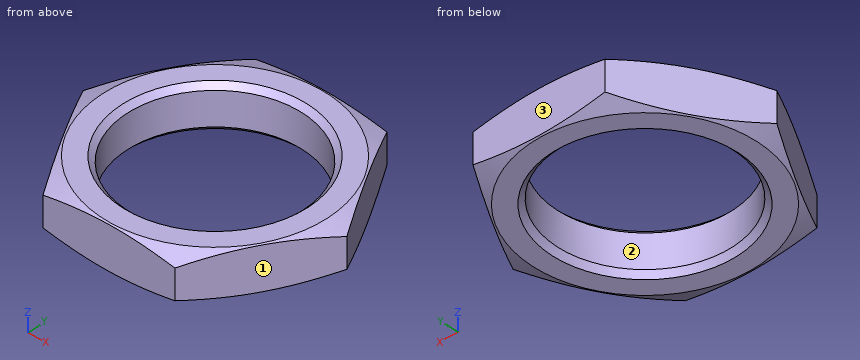
from build123d import *

# Parameters (mm, degrees)
ESQUISSE1_R        = 5
BOSS_EXTRU_1_DEPTH = 2.5
CHANFREIN1_SIZE    = 0.3


with BuildPart() as part:
    # Esquisse1 → Boss.-Extru.1 (new body)
    with BuildSketch(Plane.XY):
        Polygon((7.505553499, 0), (3.75277675, 6.5), (-3.75277675, 6.5), (-7.505553499, 0), (-3.75277675, -6.5), (3.75277675, -6.5), align=None)
        Circle(ESQUISSE1_R, mode=Mode.SUBTRACT)
    extrude(amount=BOSS_EXTRU_1_DEPTH)

    # Esquisse2 → Enlèvement de matière-Révolution1 (revolve, cut)
    with BuildSketch(Plane(origin=(0, 0, 0), x_dir=(1, 0, 0), z_dir=(0, 1, 0))):
        Polygon((-6.405553499, 0), (-7.505553499, -0.400367258), (-7.505553499, -2.099632742), (-6.405553499, -2.5), (-9.005553499, -2.5), (-9.005553499, 0), align=None)
    revolve(axis=Axis((0, 0, 0), (0, 0, 1)), mode=Mode.SUBTRACT)

    # Chanfrein1
    chanfrein1_edges = [part.edges().sort_by_distance(p)[0] for p in [
        (-5, 0, 0),
        (-5, 0, 2.5),
    ]]
    chamfer(chanfrein1_edges, length=CHANFREIN1_SIZE)


solid = part.part
Verification items for the finished model (mm, model axes). Face numbers are marked on the shaded views. Coordinates: 2 decimals unless noted, no trailing zeros. Loops run counter-clockwise (first coordinate to the right, second up) from the corner with the lowest first, then second, coordinate; pieces in that order, holes last. Notation, with made-up numbers: M 26.25,87 L 48.25,87 A32 ccw 48.25,121 Z; hole C 1,8.25 d8. An arc over 180 degrees is marked long. One line per item, written item: value.
1. Material ranges on line 1 along Y through (x, z) = (0, 1); line 2 along X through (y, z) = (1.75, 0.4); line 3 along Y through (x, z) = (4, 0.8), recorded low to high. Write a range as from..to.
Answers follow:
line 1: -6.5..-5, 5..6.5
line 2: -6.5..-4.68, 4.68..6.5
line 3: -6.07..-3, 3..6.07
2. Mould release check, pull along Y, two halves, no side actions. Record for the marked faces 1, 2 and 3: pulls with the +Y half, pulls with the -Y half, needs draft (parallel to the pull), parting line crosses it, or undercut.
Answers follow:
face 1: pulls with the -Y half
face 2: undercut
face 3: pulls with the +Y half
3. Section check A-A on x = 0. Record the cut outline in (y, z).
Answers follow:
outline: M -6.5,0.03 L -6.41,0 L -5.3,0 L -5,0.3 L -5,2.2 L -5.3,2.5 L -6.41,2.5 L -6.5,2.47 Z; M 5,0.3 L 5.3,0 L 6.41,0 L 6.5,0.03 L 6.5,2.47 L 6.41,2.5 L 5.3,2.5 L 5,2.2 Z
4. Section check B-B on z = 0.9. Record the cut outline in (x, y).
Answers follow:
outline: M -7.51,0 L -3.75,-6.5 L 3.75,-6.5 L 7.51,0 L 3.75,6.5 L -3.75,6.5 Z; hole C 0,0 d10
